```python
from build123d import *

# Parameters (mm, degrees)
SKETCH_1_W          = 450
SKETCH_1_H          = 50
SKETCH_1_R          = 3
EXTRUDE_1_DEPTH     = 2
SKETCH_2_R          = 3
CUT_EXTRUDE_1_DEPTH = 3


with BuildPart() as part:
    # Эскиз1 → Бобышка-Вытянуть1 (new body)
    with BuildSketch(Plane.XY):
        with Locations((171.141952991, -2.602230483)):
            Rectangle(SKETCH_1_W, SKETCH_1_H)
        with Locations((-5.358047009, -2.602230483)):
            Circle(SKETCH_1_R, mode=Mode.SUBTRACT)
        with Locations((27.641952991, -2.602230483)):
            Circle(SKETCH_1_R, mode=Mode.SUBTRACT)
        with Locations((74.641952991, -2.602230483)):
            Circle(SKETCH_1_R, mode=Mode.SUBTRACT)
        with Locations((107.641952991, -2.602230483)):
            Circle(SKETCH_1_R, mode=Mode.SUBTRACT)
        with Locations((154.641952991, -2.602230483)):
            Circle(SKETCH_1_R, mode=Mode.SUBTRACT)
        with Locations((187.641952991, -2.602230483)):
            Circle(SKETCH_1_R, mode=Mode.SUBTRACT)
        with Locations((234.641952991, -2.602230483)):
            Circle(SKETCH_1_R, mode=Mode.SUBTRACT)
        with Locations((267.641952991, -2.602230483)):
            Circle(SKETCH_1_R, mode=Mode.SUBTRACT)
        with Locations((314.641952991, -2.602230483)):
            Circle(SKETCH_1_R, mode=Mode.SUBTRACT)
        with Locations((347.641952991, -2.602230483)):
            Circle(SKETCH_1_R, mode=Mode.SUBTRACT)
    extrude(amount=EXTRUDE_1_DEPTH)

    # Эскиз2 → Вырез-Вытянуть1 (cut, through all)
    with BuildSketch(Plane.XY.offset(2)):
        with Locations((-41.358047009, 7.397769517)):
            Circle(SKETCH_2_R)
        with Locations(Location((-41.358047009, -12.602230483, 0), (0, 0, 180))):  # turned: the seam where the file's is
            Circle(SKETCH_2_R)
        with Locations((383.641952991, -12.602230483)):
            Circle(SKETCH_2_R)
        with Locations(Location((383.641952991, 7.397769517, 0), (0, 0, 180))):  # turned: the seam where the file's is
            Circle(SKETCH_2_R)
    extrude(amount=-CUT_EXTRUDE_1_DEPTH, mode=Mode.SUBTRACT)


solid = part.part
```
Input: part model. Units: mm. Frame: model coordinates. Round coordinates to 2 decimals unless told otherwise and drop trailing zeros. Use one line per item in the form item = value. Start each with the question number.
Item 1: Section query A-A on z = 0.7. Count the separate pieces of the cut face and the enclosed holes in it, then the cut area to 3 significant figures.
Item 2: Contact query for a flat-ended pin moving along its axis: pin 1 Ø3.5 at (x, y) = (383.64, 7.4) entering from -Z. Output: stop coordinate, or through.
Item 3: Material intervals for L1, parallel to X at y = 9, z = 1.85; L2, parallel to Y at x = 270, z = 0.35; L3, parallel to Y at x = 109, z = 0.55, sorted ascending. Write a range as from..to.
Ans:
q1.separate_pieces = 1
q1.enclosed_holes = 14
q1.area = 22,100 mm^2
q2.pin_1 = through
q3.L1 = -53.86..-43.89, -38.82..381.11, 386.18..396.14
q3.L2 = -27.6..-4.46, -0.75..22.4
q3.L3 = -27.6..-5.28, 0.07..22.4
